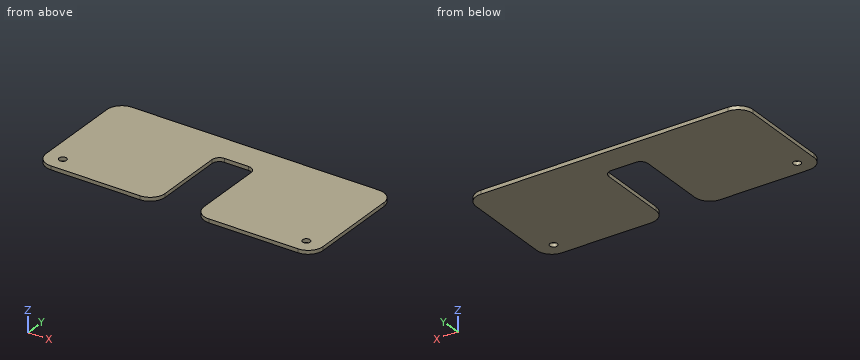
from build123d import *

# Parameters (mm, degrees)
SKETCH1_R           = 2
BOSS_EXTRUDE1_DEPTH = 2


with BuildPart() as part:
    # Sketch1 → Boss-Extrude1 (new body)
    with BuildSketch(Plane.XY):
        with BuildLine():
            Line((0, 0), (-66.5, 0))
            ThreePointArc((-66.5, 0), (-72.156854249, -2.343145751), (-74.5, -8))
            Line((-74.5, -8), (-74.5, -56))
            ThreePointArc((-74.5, -56), (-72.156854249, -61.656854249), (-66.5, -64))
            Line((-66.5, -64), (-18.5, -64))
            ThreePointArc((-18.5, -64), (-12.843145751, -61.656854249), (-10.5, -56))
            Line((-10.5, -56), (-10.5, -19))
            ThreePointArc((-10.5, -19), (-9.328427125, -16.171572875), (-6.5, -15))
            Line((-6.5, -15), (0, -15))
            Line((0, -15), (6.5, -15))
            ThreePointArc((6.5, -15), (9.328427125, -16.171572875), (10.5, -19))
            Line((10.5, -19), (10.5, -56))
            ThreePointArc((10.5, -56), (12.843145751, -61.656854249), (18.5, -64))
            Line((18.5, -64), (66.5, -64))
            ThreePointArc((66.5, -64), (72.156854249, -61.656854249), (74.5, -56))
            Line((74.5, -56), (74.5, -8))
            ThreePointArc((74.5, -8), (72.156854249, -2.343145751), (66.5, 0))
            Line((66.5, 0), (0, 0))
        make_face()
        with Locations((-65.5, -56)):
            Circle(SKETCH1_R, mode=Mode.SUBTRACT)
        with Locations(Location((65.5, -56, 0), (0, 0, 180))):
            Circle(SKETCH1_R, mode=Mode.SUBTRACT)
    extrude(amount=BOSS_EXTRUDE1_DEPTH)


solid = part.part
The model under review builds one solid part; all positions refer to its coordinate system, in mm. Give positions to 0.01 mm unless a question says otherwise; leave off trailing zeros. Order: outer loops, then holes, each group sorted by start corner. A loop starts at its lowest first (then second) coordinate and runs counter-clockwise, first axis right, second up. Notation, with made-up numbers: M 50,82.5 L 55,82.5 A19 ccw 55,109.5 Z; hole C 36,84.25 d7. An arc over 180 degrees is marked long. One line per question, with ' | ' between items. Start each with the question number.
1) Clearance check with a flat-ended pin moving along its axis: P1, Ø0.6, axis at x = -1.5, z = 1, coming from the -Y side. State where the tip first meets the part, or that it passes through.
2) Wall thickness on L1, parallel to Y at x = 65.5, z = 1.25; L2, parallel to X at y = -49, z = 0.8; L3, parallel to Y at x = 1, z = 1: over which ranges is each line inside the solid? List them lowest first. Write a range as from..to.
3) Consider section B-B, the plane z = 1.7. Give the boundary of the cut face in (x, y).
4) Consider section A-A, the plane y = -50.5. Give the boundary of the cut face in (x, z).
Found:
1) P1: stops at y = -15
2) L1: y = -64..-58, -54..0 | L2: x = -74.5..-10.5, 10.5..74.5 | L3: y = -15..0
3) outline: M -74.5,-56 A8 ccw -66.5,-64 L -18.5,-64 A8 ccw -10.5,-56 L -10.5,-19 A4 cw -6.5,-15 L 6.5,-15 A4 cw 10.5,-19 L 10.5,-56 A8 ccw 18.5,-64 L 66.5,-64 A8 ccw 74.5,-56 L 74.5,-8 A8 ccw 66.5,0 L -66.5,0 A8 ccw -74.5,-8 Z; hole C -65.5,-56 d4; hole C 65.5,-56 d4
4) outline: M -74.5,0 L -10.5,0 L -10.5,2 L -74.5,2 Z; M 10.5,0 L 74.5,0 L 74.5,2 L 10.5,2 Z
